from build123d import *

# Parameters (mm, degrees)
ESQUISSE1_R        = 2.55
BOSS_EXTRU_2_DEPTH = 8


with BuildPart() as part:
    # Esquisse1 → Boss.-Extru.2 (new body)
    with BuildSketch(Plane.XY):
        with BuildLine():
            Line((-45.5, 82.95), (-45.5, 26.95))
            Line((-45.5, 26.95), (-45.5, 25.95))
            Line((-45.5, 25.95), (-19.5, 25.95))
            Line((-19.5, 25.95), (-19.5, 30.95))
            ThreePointArc((-19.5, 30.95), (-20.671572875, 33.778427125), (-23.5, 34.95))
            Line((-23.5, 34.95), (-29.5, 34.95))
            Line((-29.5, 34.95), (-29.5, 73.95))
            Line((-29.5, 73.95), (-23.5, 73.95))
            ThreePointArc((-23.5, 73.95), (-20.671572875, 75.121572875), (-19.5, 77.95))
            Line((-19.5, 77.95), (-19.5, 82.95))
            Line((-19.5, 82.95), (-19.5, 83.95))
            Line((-19.5, 83.95), (-18.5, 83.95))
            Line((-18.5, 83.95), (18.5, 83.95))
            Line((18.5, 83.95), (19.5, 83.95))
            Line((19.5, 83.95), (19.5, 82.95))
            Line((19.5, 82.95), (19.5, 77.95))
            ThreePointArc((19.5, 77.95), (20.671572875, 75.121572875), (23.5, 73.95))
            Line((23.5, 73.95), (29.5, 73.95))
            Line((29.5, 73.95), (29.5, 34.95))
            Line((29.5, 34.95), (23.5, 34.95))
            ThreePointArc((23.5, 34.95), (20.671572875, 33.778427125), (19.5, 30.95))
            Line((19.5, 30.95), (19.5, 25.95))
            Line((19.5, 25.95), (28.5, 25.95))
            Line((28.5, 25.95), (45.5, 25.95))
            Line((45.5, 25.95), (45.5, 26.95))
            Line((45.5, 26.95), (45.5, 82.95))
            Line((45.5, 82.95), (45.5, 87.95))
            Line((45.5, 87.95), (-45.5, 87.95))
            Line((-45.5, 87.95), (-45.5, 82.95))
        make_face()
        with Locations((-23.5, 30.95)):
            Circle(ESQUISSE1_R, mode=Mode.SUBTRACT)
        with Locations((23.5, 30.95)):
            Circle(ESQUISSE1_R, mode=Mode.SUBTRACT)
        with Locations((-23.5, 77.95)):
            Circle(ESQUISSE1_R, mode=Mode.SUBTRACT)
        with Locations((23.5, 77.95)):
            Circle(ESQUISSE1_R, mode=Mode.SUBTRACT)
    extrude(amount=BOSS_EXTRU_2_DEPTH)


solid = part.part
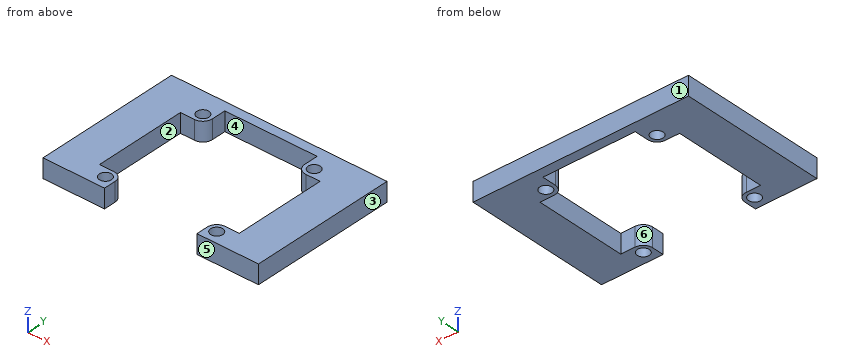
CAD build for the part. Positions are in the model's coordinates, mm. Face numbers are marked on the shaded views. A direction names the side the tool comes from. Give positions to 0.01 mm unless a question says otherwise; leave off trailing zeros. Order: outer loops, then holes, each group sorted by start corner. A loop starts at its lowest first (then second) coordinate and runs counter-clockwise, first axis right, second up. Notation, with made-up numbers: (86, 88) - (91, 88) arc R9 cw to (91, 96) - close; hole circle Ø8 at (-36, 49.5). An arc over 180 degrees is marked (long way). Answer in a Markdown table with one row per item.
1. Probe probe 1 along Y at (x, z) = (-23.5, 5.5); probe 2 along X at (y, z) = (65.5, 6). List the from-to ranges inside material, lowest first. Write a range as [from, to].
Data:
| item | result |
|---|---|
| probe 1 | y = [25.95, 28.4], [33.5, 34.95], [73.95, 75.4], [80.5, 87.95] |
| probe 2 | x = [-45.5, -29.5], [29.5, 45.5] |
2. Pull direction Y, two halves, no side cores. Call the marked faces 1, 2 and 3: pulls with the +Y half, pulls with the -Y half, needs draft (parallel to the pull), parting line crosses it, or undercut.
Data:
| item | result |
|---|---|
| face 1 | pulls with the +Y half |
| face 2 | undercut |
| face 3 | needs draft |
3. Flat gauge pins, fed straight in: pin 1 (4 mm diameter, centred on x = 2.5, z = 4, fed in from -Y); pin 2 (3 mm diameter, centred on x = 23.5, y = 30.95, fed in from +Z); pin 3 (6.5 mm diameter, centred on x = -23.5, y = 77.95, fed in from -Z). Where does each tip first touch, or does it go through?
Data:
| item | result |
|---|---|
| pin 1 | stops at y = 83.95 |
| pin 2 | passes through |
| pin 3 | stops at z = 0 |
4. Tool access for the marked faces 4, 5 and 6: list every direction of +Z, -Z, +X, -X, +Y, -Y with a clear straight run to the whole face (end or side of a thin tool).
Data:
| item | result |
|---|---|
| face 4 | +Z, -Z, -Y |
| face 5 | +Z, -Z, +X, -X, -Y |
| face 6 | +Z, -Z |
5. Saw through at C-C, the plane x = 17.5. Give the cut face in (y, z), plus the area to 3 significant figures.
Data:
| item | result |
|---|---|
| outline | (83.95, 0) - (87.95, 0) - (87.95, 8) - (83.95, 8) - close |
| area | 32.0 mm² |
6. Saw through at A-A, the plane z = 1.75. Give the cut face in (x, y).
Data:
| item | result |
|---|---|
| outline | (-45.5, 25.95) - (-19.5, 25.95) - (-19.5, 30.95) arc R4 ccw to (-23.5, 34.95) - (-29.5, 34.95) - (-29.5, 73.95) - (-23.5, 73.95) arc R4 ccw to (-19.5, 77.95) - (-19.5, 83.95) - (19.5, 83.95) - (19.5, 77.95) arc R4 ccw to (23.5, 73.95) - (29.5, 73.95) - (29.5, 34.95) - (23.5, 34.95) arc R4 ccw to (19.5, 30.95) - (19.5, 25.95) - (45.5, 25.95) - (45.5, 87.95) - (-45.5, 87.95) - close; hole circle Ø5.1 at (-23.5, 30.95); hole circle Ø5.1 at (-23.5, 77.95); hole circle Ø5.1 at (23.5, 30.95); hole circle Ø5.1 at (23.5, 77.95) |
7. Saw through at B-B, the plane y = 79.5. Give the cut face in (x, z), plus the area to 3 significant figures.
Data:
| item | result |
|---|---|
| outline | (-45.5, 0) - (-25.52, 0) - (-25.52, 8) - (-45.5, 8) - close; (-21.48, 0) - (-19.5, 0) - (-19.5, 8) - (-21.48, 8) - close; (19.5, 0) - (21.48, 0) - (21.48, 8) - (19.5, 8) - close; (25.52, 0) - (45.5, 0) - (45.5, 8) - (25.52, 8) - close |
| area | 351 mm² |
